Input: part model. Units: mm. Frame: model coordinates. A direction names the side the tool comes from. Round coordinates to 2 decimals unless told otherwise and drop trailing zeros. Order: outer loops, then holes, each group sorted by start corner. A loop starts at its lowest first (then second) coordinate and runs counter-clockwise, first axis right, second up. Notation, with made-up numbers: (12, 79) -> (53, 79) arc R5 cw to (53, 88) -> close; hole circle Ø8 at (-28.75, 25.25). An arc over 180 degrees is marked (long way). Use a Markdown table: item, result.
from build123d import *

# Parameters (mm, degrees)
SKETCH_1_W          = 15
SKETCH_1_H          = 15
SKETCH_1_W_2        = 13
SKETCH_1_H_2        = 13
EXTRUDE_1_DEPTH     = 665
SKETCH_3_R          = 1.45
CUT_EXTRUDE_1_DEPTH = 666.211432554
SKETCH_4_R          = 1.45
CUT_EXTRUDE_2_DEPTH = 666.211432554


with BuildPart() as part:
    # 草图1 → 凸台-拉伸1 (new body)
    with BuildSketch(Plane(origin=(0, 0, 0), x_dir=(0, 0, -1), z_dir=(1, 0, 0))):
        Rectangle(SKETCH_1_W, SKETCH_1_H)
        Rectangle(SKETCH_1_W_2, SKETCH_1_H_2, mode=Mode.SUBTRACT)
    extrude(amount=EXTRUDE_1_DEPTH)

    # 草图3 → 切除-拉伸1 (cut, through all)
    with BuildSketch(Plane(origin=(0, 0, -7.5), x_dir=(-1, 0, 0), z_dir=(0, 0, -1))):
        with Locations((-9, 0)):
            Circle(SKETCH_3_R)
        with Locations((-19, 0)):
            Circle(SKETCH_3_R)
        with Locations((-440, 0)):
            Circle(SKETCH_3_R)
        with Locations((-450, 0)):
            Circle(SKETCH_3_R)
    extrude(amount=-CUT_EXTRUDE_1_DEPTH, mode=Mode.SUBTRACT)

    # 草图4 → 切除-拉伸2 (cut, through all)
    with BuildSketch(Plane(origin=(0, 7.5, 0), x_dir=(1, 0, 0), z_dir=(0, 1, 0))):
        with Locations(Location((630, 0, 0), (0, 0, 270))):
            Circle(SKETCH_4_R)
        with Locations(Location((640, 0, 0), (0, 0, 270))):
            Circle(SKETCH_4_R)
        with Locations(Location((14, 0, 0), (0, 0, 270))):
            Circle(SKETCH_4_R)
        with Locations(Location((24, 0, 0), (0, 0, 270))):
            Circle(SKETCH_4_R)
        with Locations(Location((64, 0, 0), (0, 0, 270))):
            Circle(SKETCH_4_R)
        with Locations(Location((104, 0, 0), (0, 0, 270))):
            Circle(SKETCH_4_R)
        with Locations(Location((340, 0, 0), (0, 0, 270))):
            Circle(SKETCH_4_R)
        with Locations(Location((400, 0, 0), (0, 0, 270))):
            Circle(SKETCH_4_R)
        with Locations(Location((460, 0, 0), (0, 0, 270))):
            Circle(SKETCH_4_R)
    extrude(amount=-CUT_EXTRUDE_2_DEPTH, mode=Mode.SUBTRACT)


solid = part.part
1) Cut plane A-A on x = 267. Return loops of the section in (y, z), and give its area (3 significant figures).
Results found:
| item | result |
|---|---|
| outline | (-7.5, -7.5) -> (7.5, -7.5) -> (7.5, 7.5) -> (-7.5, 7.5) -> close; hole (-6.5, -6.5) -> (6.5, -6.5) -> (6.5, 6.5) -> (-6.5, 6.5) -> close |
| area | 56.0 mm² |
2) Pin query (flat end, axial travel): pin 1 Ø2.5 at (x, z) = (630, 0) entering from +Y. Return the tip coordinate at first contact, or that it passes through.
Results found:
| item | result |
|---|---|
| pin 1 | passes through |
3) Line query: L1, parallel to Y at x = 331, z = 1; L2, parallel to Z at x = 64, y = 7.1. Output: solid intervals per line, ascending. Write a range as [from, to].
Results found:
| item | result |
|---|---|
| L1 | y = [-7.5, -6.5], [6.5, 7.5] |
| L2 | z = [-7.5, -1.45], [1.45, 7.5] |
4) Set-up query: faces 1 (the flat face through (328, 0, 6.5)), 2 (the flat face through (0, 0, 7)). Return all of +Z, -Z, +X, -X, +Y, -Y with unobstructed straight access to the full face (end or side cutting, diameter ignored); none if empty.
Results found:
| item | result |
|---|---|
| face 1 | +X, -X |
| face 2 | +Z, -Z, -X, +Y, -Y |
5) Pull-direction query (Y, two-part tool) for faces 3 (the flat face through (328, 6.5, 0)), 4 (the flat face through (328, 0, 7.5)), 5 (the flat face through (328, 7.5, 0)); classes: +Y half, -Y half, draft (parallel to the pull), parting line (faces both ways), or undercut.
Results found:
| item | result |
|---|---|
| face 3 | undercut |
| face 4 | draft |
| face 5 | +Y half |
